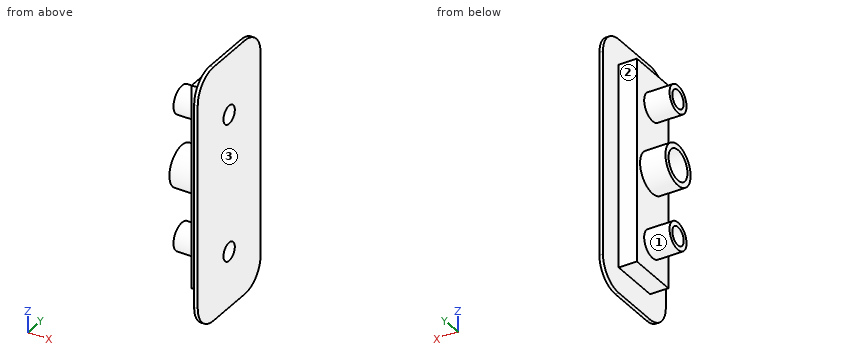
```python
from build123d import *
from build123d.topology import SkipClean

# Parameters (mm, degrees)
SKETCH1_R                = 4
SKETCH1_R_2              = 3
BOSS_EXTRUDE1_DEPTH      = 5
SKETCH2_W                = 40
SKETCH2_H                = 10
SKETCH2_R                = 3
BOSS_EXTRUDE2_DEPTH      = 3.6
SKETCH7_W                = 50
SKETCH7_H                = 20
BOSS_EXTRUDE3_DEPTH      = 0.7
M3_CLEARANCE_HOLE1_D     = 3.6
M3_CLEARANCE_HOLE1_DEPTH = 12
M3_CLEARANCE_HOLE1_TIP   = 1.081549114
SKETCH8_R                = 2.7
SKETCH8_R_2              = 1.8
BOSS_EXTRUDE4_DEPTH      = 5
FILLET2_R                = 5


with BuildPart() as part:
    # Sketch1 → Boss-Extrude1 (new body)
    with BuildSketch(Plane(origin=(0, 0, 0), x_dir=(0, 0, -1), z_dir=(1, 0, 0))):
        Circle(SKETCH1_R)
        Circle(SKETCH1_R_2, mode=Mode.SUBTRACT)
    extrude(amount=BOSS_EXTRUDE1_DEPTH)

    # Sketch2 → Boss-Extrude2 (add)
    with BuildSketch(Plane(origin=(5, 0, 0), x_dir=(0, 0, -1), z_dir=(1, 0, 0))):
        Rectangle(SKETCH2_W, SKETCH2_H)
        Circle(SKETCH2_R, mode=Mode.SUBTRACT)
    extrude(amount=BOSS_EXTRUDE2_DEPTH)

    # Sketch7 → Boss-Extrude3 (add)
    with BuildSketch(Plane(origin=(8.6, 0, 0), x_dir=(0, 0, -1), z_dir=(1, 0, 0))):
        Rectangle(SKETCH7_W, SKETCH7_H)
    extrude(amount=BOSS_EXTRUDE3_DEPTH)

    # M3 Clearance Hole1
    with Locations(Plane.ZY.offset(-5)):
        with Locations((-14, 0), (13, 0)):
            Hole(M3_CLEARANCE_HOLE1_D / 2, depth=M3_CLEARANCE_HOLE1_DEPTH)
            with Locations((0, 0, -(M3_CLEARANCE_HOLE1_DEPTH + M3_CLEARANCE_HOLE1_TIP / 2))):  # 118° drill point
                Cone(0, M3_CLEARANCE_HOLE1_D / 2, M3_CLEARANCE_HOLE1_TIP, mode=Mode.SUBTRACT)

    # Sketch8 → Boss-Extrude4 (add)
    # profile 1 of 2: a face of its own
    with SkipClean():  # the faces are left unmerged after this step: merging them gives an invalid solid
        with BuildSketch(Plane.ZY.offset(-5)):
            with Locations((-14, 0)):
                Circle(SKETCH8_R)
            with Locations((-14, 0)):
                Circle(SKETCH8_R_2, mode=Mode.SUBTRACT)
        # profile 2 of 2: a face of its own
        with BuildSketch(Plane.ZY.offset(-5)):
            with Locations((13, 0)):
                Circle(SKETCH8_R)
            with Locations((13, 0)):
                Circle(SKETCH8_R_2, mode=Mode.SUBTRACT)
        extrude(amount=BOSS_EXTRUDE4_DEPTH)
    add(part.part.scale(1), mode=Mode.REPLACE)  # the faces are merged on a copy

    # Fillet2
    fillet2_edges = [part.edges().sort_by_distance(p)[0] for p in [
        (8.95, 10, 25),
        (8.95, -10, 25),
        (8.95, -10, -25),
        (8.95, 10, -25),
    ]]
    fillet(fillet2_edges, radius=FILLET2_R)


solid = part.part
```
Geometry check sheet. Reference: the model listing, model coordinates, mm. Face numbers are marked on the shaded views. A direction names the side the tool comes from. Round coordinates to 2 decimals unless told otherwise and drop trailing zeros. Loops run counter-clockwise (first coordinate to the right, second up) from the corner with the lowest first, then second, coordinate; pieces in that order, holes last. Notation, with made-up numbers: (7, 66.25) - (65, 66.25) arc R19 ccw to (65, 74.25) - close; hole circle Ø2 at (54, 29.25). An arc over 180 degrees is marked (long way). Write item = value, one per line. Start each with the question number.
1. Thickness scan on line 1 (Y direction, x = 2.7, z = 13); line 2 (Y direction, x = 6.8, z = 13); line 3 (X direction, y = -2.5, z = -11). Record the ranges inside material, lowest first.
2. Set-up check for the marked faces 1, 2 and 3: record each of +Z, -Z, +X, -X, +Y, -Y from which the full face is reachable in a straight line by a thin tool's end or side.
3. Section check B-B on z = -14. Enter the section's corners in (x, y).
4. Section check D-D on z = 0. Enter the section's corners in (x, y), then the cut area to 3 significant figures.
5. Depth check by flat-ended pin: pin 1 (4 mm diameter, centred on x = 1.5, z = 7.5, fed in from +Y); pin 2 (1.1 mm diameter, centred on x = 6.5, y = -1.5, fed in from -Z); pin 3 (5 mm diameter, centred on x = 7, y = -6.5, fed in from +Z); pin 4 (3 mm diameter, centred on x = 5, y = 6, fed in from +Z). Enter the tip coordinate at first touch or a pass-through.
6. Section check A-A on y = 0. Give the number of separate pieces and of enclosed holes in the cut face, then the cut area to 3 significant figures.
7. Section check C-C on x = 4. Enter the section's corners in (y, z).
Working result:
q1.line_1 = -2.7 to -1.8, 1.8 to 2.7
q1.line_2 = -5 to -1.8, 1.8 to 5
q1.line_3 = 5 to 9.3
q2.face_1 = -X
q2.face_2 = +Z, -Z, -X, +Y
q2.face_3 = +Z, -Z, +X, +Y, -Y
q3.outline = (0, -2.7) - (5, -2.7) - (5, -5) - (8.6, -5) - (8.6, -10) - (9.3, -10) - (9.3, -1.8) - (0, -1.8) - close; (0, 1.8) - (9.3, 1.8) - (9.3, 10) - (8.6, 10) - (8.6, 5) - (5, 5) - (5, 2.7) - (0, 2.7) - close
q4.outline = (0, -4) - (5, -4) - (5, -5) - (8.6, -5) - (8.6, -10) - (9.3, -10) - (9.3, 10) - (8.6, 10) - (8.6, 5) - (5, 5) - (5, 4) - (0, 4) - (0, 3) - (8.6, 3) - (8.6, -3) - (0, -3) - close
q4.area = 38.4 mm^2
q5.pin_1 = through
q5.pin_2 = -20
q5.pin_3 = 25
q5.pin_4 = 20
q6.separate_pieces = 3
q6.enclosed_holes = 0
q6.area = 154 mm^2
q7.outline = circle Ø8 at (0, 0); circle Ø5.4 at (0, -14); circle Ø5.4 at (0, 13); hole circle Ø6 at (0, 0); hole circle Ø3.6 at (0, -14); hole circle Ø3.6 at (0, 13)
